from build123d import *

# Parameters (mm, degrees)
BOSS_EXTRUDE1_DEPTH      = 6
BOSS_EXTRUDE1_DEPTH_BACK = 6
SKETCH1_W                = 16.7
SKETCH1_H                = 3
SKETCH1_R                = 1.1
SKETCH2_W                = 3
SKETCH2_H                = 11
SKETCH2_W_2              = 9
SKETCH2_H_2              = 8
SKETCH2_W_3              = 7.8
SKETCH2_H_3              = 2
CUT_EXTRUDE1_DEPTH       = 5


with BuildPart() as part:
    # Sketch1 → Boss-Extrude1 (new, two sides: drawn at the far end of the back side and taken through both)
    with BuildSketch(Plane.XY.offset(-BOSS_EXTRUDE1_DEPTH_BACK)):
        Rectangle(SKETCH1_W, SKETCH1_H)
        with Locations((-6.75, 0)):
            Circle(SKETCH1_R, mode=Mode.SUBTRACT)
        with Locations((6.75, 0)):
            Circle(SKETCH1_R, mode=Mode.SUBTRACT)
    extrude(amount=BOSS_EXTRUDE1_DEPTH + BOSS_EXTRUDE1_DEPTH_BACK)

    # Sketch2 → Cut-Extrude1 (cut)
    with BuildSketch(Plane(origin=(0, 1.5, 0), x_dir=(1, 0, 0), z_dir=(0, 1, 0))):
        Rectangle(SKETCH2_W, SKETCH2_H)
        with Locations((8.35, -6)):
            Rectangle(SKETCH2_W_2, SKETCH2_H_2)
        with Locations((8.35, 6)):
            Rectangle(SKETCH2_W_2, SKETCH2_H_2)
        with Locations((-8.35, 0)):
            Rectangle(SKETCH2_W_3, SKETCH2_H_3)
    extrude(amount=-CUT_EXTRUDE1_DEPTH, mode=Mode.SUBTRACT)


solid = part.part
For this review, take the finished solid that the model builds, in its own axes (mm). A direction names the side the tool comes from. Coordinates: 2 decimals unless noted, no trailing zeros. Order: outer loops, then holes, each group sorted by start corner. A loop starts at its lowest first (then second) coordinate and runs counter-clockwise, first axis right, second up. Notation, with made-up numbers: (48.5, -4.75) - (63.5, -4.75) arc R20 ccw to (63.5, 21.25) - close; hole circle Ø11 at (-30, 12). An arc over 180 degrees is marked (long way). Answer as CSV lines item,"result". Start each with the question number.
1) Machinability: for faces 4 (the flat face through (-1.5, 0, 0)), 5 (the flat face through (-5.6, 0.7, -1)), 6 (the flat face through (3.85, 0, -4)), which of the approach directions +Z, -Z, +X, -X, +Y, -Y give a long, thin tool a straight path to every point of the face, cutting with its end or side? Answer none if there is none.
2) Add section B-B (x = -0.25). State the section outline as (y, z) points, then the cut area to 3 significant figures.
3) Draft analysis for pull direction X (two halves, no side actions). For faces 1 (the flat face through (1.5, 0, 0)), 2 (the flat face through (-8.35, 0, 3)), 3 (the flat face through (8.35, 0, 0)), state which applies: +X half, -X half, draft (parallel to the pull), parting line (faces both ways), or undercut.
4) Add section A-A (z = 5). State the section outline as (x, y) points.
5) Insertion check: P1, Ø0.9, axis at y = -0.5, z = 4.5, coming from the +X side; P2, Ø0.6, axis at y = 0.5, z = 0, coming from the -X side; P3, Ø1.5, axis at x = 5.5, y = 0, coming from the +Z side. Each pin has a flat end and moves straight along its axis. Give the tip position at first contact, or say it passes through.
6) To check wall thickness, follow line 1 along X through (y, z) = (0, 3.4); line 2 along X through (y, z) = (0, -0.3); line 3 along X through (y, z) = (1.35, -2.75). State the ranges of each line that lie inside material, in increasing order. Write a range as [from, to].
7) Add section D-D (x = -6.75). State the section outline as (y, z) points, then the cut area to 3 significant figures.
8) Add section C-C (y = 0). State the section outline as (x, z) points, then the cut area to 3 significant figures.
Result:
1,face 4,"+Y, -Y"
1,face 5,"-X, +Y, -Y"
1,face 6,"-Z, +X, +Y, -Y"
2,outline,"(-1.5, -6) - (1.5, -6) - (1.5, -5.5) - (-1.5, -5.5) - close; (-1.5, 5.5) - (1.5, 5.5) - (1.5, 6) - (-1.5, 6) - close"
2,area,"3.00 mm^2"
3,face 1,"undercut"
3,face 2,"-X half"
3,face 3,"+X half"
4,outline,"(-8.35, -1.5) - (-1.5, -1.5) - (-1.5, 1.5) - (-8.35, 1.5) - close; (1.5, -1.5) - (3.85, -1.5) - (3.85, 1.5) - (1.5, 1.5) - close; hole circle Ø2.2 at (-6.75, 0)"
5,P1,"x = 3.85"
5,P2,"x = -4.45"
5,P3,"z = 2"
6,line 1,"[-8.35, -7.85], [-5.65, -1.5], [1.5, 3.85]"
6,line 2,"[-4.45, -1.5], [1.5, 5.65], [7.85, 8.35]"
6,line 3,"[-8.35, -1.5], [1.5, 3.85]"
7,outline,"(-1.5, -6) - (-1.1, -6) - (-1.1, -1) - (-1.5, -1) - close; (-1.5, 1) - (-1.1, 1) - (-1.1, 6) - (-1.5, 6) - close; (1.1, -6) - (1.5, -6) - (1.5, -1) - (1.1, -1) - close; (1.1, 1) - (1.5, 1) - (1.5, 6) - (1.1, 6) - close"
7,area,"8.00 mm^2"
8,outline,"(-8.35, -6) - (-7.85, -6) - (-7.85, -1) - (-8.35, -1) - close; (-8.35, 1) - (-7.85, 1) - (-7.85, 6) - (-8.35, 6) - close; (-5.65, -6) - (3.85, -6) - (3.85, -2) - (5.65, -2) - (5.65, 2) - (3.85, 2) - (3.85, 6) - (-5.65, 6) - (-5.65, 1) - (-4.45, 1) - (-4.45, -1) - (-5.65, -1) - close; (7.85, -2) - (8.35, -2) - (8.35, 2) - (7.85, 2) - close; hole (-1.5, -5.5) - (1.5, -5.5) - (1.5, 5.5) - (-1.5, 5.5) - close"
8,area,"92.8 mm^2"
